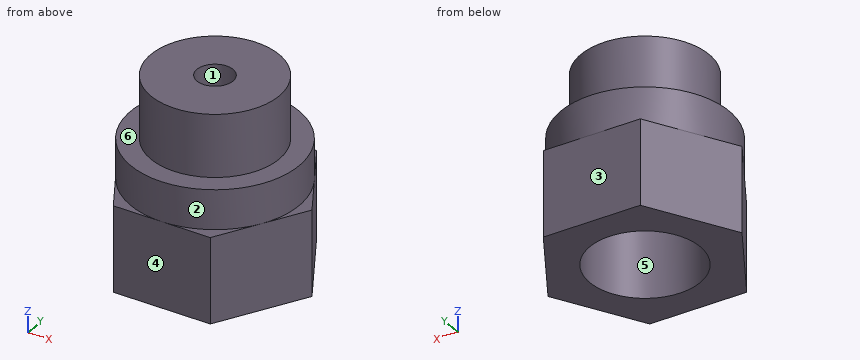
from build123d import *

# Parameters (mm, degrees)
BOSS_EXTRUDE1_DEPTH = 6.5
SKETCH2_R           = 6.4
BOSS_EXTRUDE2_DEPTH = 3
SKETCH3_R           = 4.2
CUT_EXTRUDE1_DEPTH  = 7.5
SKETCH5_R           = 4.875
BOSS_EXTRUDE3_DEPTH = 4.75
SKETCH6_R           = 1.375
CUT_EXTRUDE2_DEPTH  = 18.281083106


with BuildPart() as part:
    # Sketch1 → Boss-Extrude1 (new body)
    with BuildSketch(Plane.XY):
        Polygon((7.390083446, 0), (3.695041723, 6.4), (-3.695041723, 6.4), (-7.390083446, 0), (-3.695041723, -6.4), (3.695041723, -6.4), align=None)
    extrude(amount=BOSS_EXTRUDE1_DEPTH)

    # Sketch2 → Boss-Extrude2 (add)
    with BuildSketch(Plane.XY.offset(6.5)):
        with Locations(Location((0, 0, 0), (0, 0, 150))):
            Circle(SKETCH2_R)
    extrude(amount=BOSS_EXTRUDE2_DEPTH)

    # Sketch3 → Cut-Extrude1 (cut)
    with BuildSketch(Plane(origin=(0, 0, 0), x_dir=(-1, 0, 0), z_dir=(0, 0, -1))):
        Circle(SKETCH3_R)
    extrude(amount=-CUT_EXTRUDE1_DEPTH, mode=Mode.SUBTRACT)

    # Sketch5 → Boss-Extrude3 (add)
    with BuildSketch(Plane.XY.offset(9.5)):
        Circle(SKETCH5_R)
    extrude(amount=BOSS_EXTRUDE3_DEPTH)

    # Sketch6 → Cut-Extrude2 (cut, through all)
    with BuildSketch(Plane.XY.offset(14.25)):
        Circle(SKETCH6_R)
    extrude(amount=-CUT_EXTRUDE2_DEPTH, mode=Mode.SUBTRACT)


solid = part.part
The model under review builds one solid part; all positions refer to its coordinate system, in mm. Face numbers are marked on the shaded views. A direction names the side the tool comes from. Round coordinates to 2 decimals unless told otherwise and drop trailing zeros. Write each loop counter-clockwise with the first axis right and the second up, starting at its lowest first coordinate (ties: lowest second). Pieces come first, ordered by that corner, then holes. Notation, with made-up numbers: (25, -21) - (77, -21) arc R29 ccw to (77, 2) - close; hole circle Ø8 at (44, 72). An arc over 180 degrees is marked (long way). One line per item, written item: value. Start each with the question number.
1. Machinability: for the marked faces 4, 5 and 6, which of the approach directions +Z, -Z, +X, -X, +Y, -Y give a long, thin tool a straight path to every point of the face, cutting with its end or side? Answer none if there is none.
2. Clearance check with flat-ended pins moving along their axes: P1, Ø5, axis at y = 3, z = 6, coming from the -X side; P2, Ø5, axis at x = 0, y = 0, coming from the -Z side; P3, Ø0.9, axis at x = 7, y = -1.5, coming from the +Z side. State where each tip first meets the part, or that it passes through.
3. Consider section D-D on y = 0.25. Write out the cut boundary in (x, z), and give its area (3 significant figures).
4. To check wall thickness, follow L1, parallel to Y at x = 0, z = 2.75; L2, parallel to Y at x = 0, z = 11 (3 decimals); L3, parallel to Z at x = 4.75, y = -4.25. State the ranges of each line that lie inside material, in increasing order. Write a range as from..to.
5. Consider section C-C on y = 2.5. Write out the cut boundary in (x, z).
6. The part is to be moulded in two halves that separate along X. For the marked faces 1, 2 and 3, say which applies: released by +X, released by -X, zero draft, split by the parting line, or undercut.
7. Consider section A-A on z = 4.75. Write out the cut boundary in (x, y), and give its area (3 significant figures).
Checks:
1. face 4: +Z, -Z, +X, -X, -Y
1. face 5: -Z
1. face 6: +Z
2. P1: stops at x = -7.1
2. P2: stops at z = 7.5
2. P3: stops at z = 6.5
3. outline: (-7.25, 0) - (-4.19, 0) - (-4.19, 7.5) - (-1.35, 7.5) - (-1.35, 14.25) - (-4.87, 14.25) - (-4.87, 9.5) - (-6.4, 9.5) - (-6.4, 6.5) - (-7.25, 6.5) - close; (1.35, 7.5) - (4.19, 7.5) - (4.19, 0) - (7.25, 0) - (7.25, 6.5) - (6.4, 6.5) - (6.4, 9.5) - (4.87, 9.5) - (4.87, 14.25) - (1.35, 14.25) - close
3. area: 97.7 mm^2
4. L1: y = -6.4..-4.2, 4.2..6.4
4. L2: y = -4.875..-1.375, 1.375..4.875
4. L3: z = 0..9.5
5. outline: (-5.95, 0) - (-3.37, 0) - (-3.37, 7.5) - (3.37, 7.5) - (3.37, 0) - (5.95, 0) - (5.95, 6.5) - (5.89, 6.5) - (5.89, 9.5) - (4.19, 9.5) - (4.19, 14.25) - (-4.19, 14.25) - (-4.19, 9.5) - (-5.89, 9.5) - (-5.89, 6.5) - (-5.95, 6.5) - close
6. face 1: undercut
6. face 2: split by the parting line
6. face 3: zero draft
7. outline: (-7.39, 0) - (-3.7, -6.4) - (3.7, -6.4) - (7.39, 0) - (3.7, 6.4) - (-3.7, 6.4) - close; hole circle Ø8.4 at (0, 0)
7. area: 86.5 mm^2
